from build123d import *

# Parameters (mm, degrees)
CUT_EXTRUDE_1_DEPTH = 5


with BuildPart() as part:
    # 草图1 → 旋转1 (revolve)
    with BuildSketch(Plane.XY, mode=Mode.PRIVATE) as revolve_1_sk:
        Polygon((10, 0), (10, 3.5), (9.5, 4), (9, 3.5), (8.5, 4), (8, 3.5), (7.5, 4), (7, 3.5), (6.5, 4), (6, 3.5), (5.5, 4), (5, 3.5), (4.5, 4), (4, 3.5), (3.5, 4), (3, 3.5), (2.5, 4), (2, 3.5), (1.5, 4), (1, 3.5), (0.5, 4), (0, 3.5), (0, 0), align=None)
    revolve(revolve_1_sk.sketch.rotate(Axis((0.5, 0, 0), (1, 0, 0)), 90), axis=Axis((0.5, 0, 0), (1, 0, 0)))

    # 草图3 → 切除-拉伸1 (cut)
    with BuildSketch(Plane(origin=(10, 0, 0), x_dir=(0, 0, -1), z_dir=(1, 0, 0))):
        Polygon((2.886751346, 0), (1.443375673, 2.5), (-1.443375673, 2.5), (-2.886751346, 0), (-1.443375673, -2.5), (1.443375673, -2.5), align=None)
    extrude(amount=-CUT_EXTRUDE_1_DEPTH, mode=Mode.SUBTRACT)


solid = part.part
Model file for the job. Use its own axes, mm. Give positions to 0.01 mm unless a question says otherwise; leave off trailing zeros. Loops run counter-clockwise (first coordinate to the right, second up) from the corner with the lowest first, then second, coordinate; pieces in that order, holes last.
Item 1: Mould opens along Y. For faces 1 (the face through (7.535, -1.267, -2.155)), 2 (the face through (8, 2.5, 0)) say: +Y half, -Y half, draft (parallel to the pull), parting line (faces both ways), or undercut.
Check values:
face 1: undercut
face 2: undercut
Item 2: Slice it at A-A (x = 5.75). Write the cut outline in (y, z).
Check values:
outline: circle Ø7.5 at (0, 0); hole (-2.5, -1.44) - (0, -2.89) - (2.5, -1.44) - (2.5, 1.44) - (0, 2.89) - (-2.5, 1.44) - close
Item 3: Drill centre lines: line 1 along X through (y, z) = (-1, 2); line 2 along Z through (x, y) = (3.75, -2); line 3 along Z through (x, y) = (4.75, 0.5). Where is each one in solid material? Low to high.
Check values:
line 1: x = 0 to 5
line 2: z = -3.17 to 3.17
line 3: z = -3.72 to 3.72
Item 4: Drop flat-ended pins along their axis: P1, Ø1, axis at x = 5.5, z = -3, coming from the +Y side; P2, Ø2.5, axis at y = 0.5, z = 0.5, coming from the +X side; P3, Ø2, axis at x = 8, y = -1, coming from the +Z side. Give the stop position or say it passes through.
Check values:
P1: stops at y = 3.12
P2: stops at x = 5
P3: stops at z = 4
Item 5: Slice it at B-B (x = 4.75). Write the cut outline in (y, z), plus the area to 3 significant figures.
Check values:
outline: circle Ø7.5 at (0, 0)
area: 44.2 mm2
